Work out the finished part from the listing and answer in its coordinate system (mm). A direction names the side the tool comes from. Coordinates: 2 decimals unless noted, no trailing zeros. Write each loop counter-clockwise with the first axis right and the second up, starting at its lowest first coordinate (ties: lowest second). Pieces come first, ordered by that corner, then holes. Notation, with made-up numbers: (35.5, 13) - (87.5, 13) arc R14 ccw to (87.5, 26) - close; hole circle Ø7 at (42, 88). An arc over 180 degrees is marked (long way). Use one line per item in the form item = value. Start each with the question number.
Item 1: A cutting plane is placed at A-A (x = -11.4). Write down the section's boundary in (y, z) (3 decimals).
Item 2: Given pin 1 (4.5 mm diameter, centred on x = -10.5, z = 5, fed in from +Y); pin 2 (0.9 mm diameter, centred on y = 1, z = 4, fed in from -X); pin 3 (1.5 mm diameter, centred on y = 4, z = -9.5, fed in from +X), each flat-ended and moving along its own axis, determine where each tip first touches the part or whether it passes through.
Item 3: A cutting plane is placed at B-B (z = 9.5). Write down the section's boundary in (x, y).
Item 4: Determine the mould class of faces 3 (the flat face through (-19.6, -2, 0)), 4 (the flat face through (-3.2, -2, 0)), 5 (the flat face through (-9, -3.2, 3)) for opening direction X: released by +X, released by -X, zero draft, split by the parting line, or undercut.
Item 5: Consider probe 1 along X at (y, z) = (-0.85, 0) (3 decimals); probe 2 along Z at (x, y) = (-11.4, -2.6) (3 decimals); probe 3 along X at (y, z) = (-1.3, 0) (3 decimals). Determine where each line is inside the solid, lowest interval first.
Item 6: A cutting plane is placed at C-C (y = 2.75). Write down the section's boundary in (x, z), then the cut area to 3 significant figures.
Item 7: For faces 1 (the flat face through (-7, -0.66, 0)), 2 (the flat face through (-5, 0, 12.7)), determine the directions among +Z, -Z, +X, -X, +Y, -Y from which every point of the face is accessible in a straight line to the end or side of a thin tool.
Item 8: A cutting plane is placed at D-D (z = 1.5). Write down the section's boundary in (x, y), then the cut area to 3 significant figures.
from build123d import *

# Parameters (mm, degrees)
BASE_EXTRUDE_DEPTH = 12.7
SKETCH9_R          = 3.175
CUT_EXTRUDE1_DEPTH = 26.007470884


with BuildPart() as part:
    # Sketch1 → Base-Extrude (new, symmetric)
    with BuildSketch(Plane.XY):
        with BuildLine():
            Line((-14.52, -0.66), (-5.74, -0.66))
            Line((-5.74, -0.66), (-5.74, 0))
            ThreePointArc((-5.74, 0), (0, 5.74), (5.74, 0))
            Line((5.74, 0), (5.74, 1.88))
            ThreePointArc((5.74, 1.88), (7.536051224, -2.456051224), (3.2, -0.66))
            Line((3.2, -0.66), (3.2, 0))
            ThreePointArc((3.2, 0), (0, 3.2), (-3.2, 0))
            Line((-3.2, 0), (-3.2, -3.2))
            Line((-3.2, -3.2), (-19.6, -3.2))
            Line((-19.6, -3.2), (-19.6, -0.66))
            ThreePointArc((-19.6, -0.66), (-17.06, 1.88), (-14.52, -0.66))
        make_face()
    extrude(amount=BASE_EXTRUDE_DEPTH, both=True)

    # Sketch9 → Cut-Extrude1 (cut, through all)
    with BuildSketch(Plane.XZ.offset(3.2)):
        with Locations((-11.4, 0)):
            Circle(SKETCH9_R)
    extrude(amount=-CUT_EXTRUDE1_DEPTH, mode=Mode.SUBTRACT)


solid = part.part
Answer:
q1.outline = (-3.2, -12.7) - (-0.66, -12.7) - (-0.66, -3.175) - (-3.2, -3.175) - close; (-3.2, 3.175) - (-0.66, 3.175) - (-0.66, 12.7) - (-3.2, 12.7) - close
q2.pin_1 = -0.66
q2.pin_2 = -19.29
q2.pin_3 = 4.73
q3.outline = (-19.6, -3.2) - (-3.2, -3.2) - (-3.2, 0) arc R3.2 cw to (3.2, 0) - (3.2, -0.66) arc R2.54 ccw (long way) to (5.74, 1.88) - (5.74, 0) arc R5.74 ccw to (-5.74, 0) - (-5.74, -0.66) - (-14.52, -0.66) arc R2.54 ccw to (-19.6, -0.66) - close
q4.face_3 = released by -X
q4.face_4 = undercut
q4.face_5 = zero draft
q5.probe_1 = -19.6 to -14.575, -8.225 to -3.2, 3.207 to 8.273
q5.probe_2 = -12.7 to -3.175, 3.175 to 12.7
q5.probe_3 = -19.6 to -14.575, -8.225 to -3.2, 3.282 to 8.198
q6.outline = (-5.04, -12.7) - (-1.64, -12.7) - (-1.64, 12.7) - (-5.04, 12.7) - close; (1.64, -12.7) - (5.04, -12.7) - (5.04, 12.7) - (1.64, 12.7) - close
q6.area = 173 mm²
q7.face_1 = +Z, -Z, +Y
q7.face_2 = +Z, +X, -X, +Y, -Y
q8.outline = (-19.6, -3.2) - (-14.2, -3.2) - (-14.2, -0.66) - (-14.52, -0.66) arc R2.54 ccw to (-19.6, -0.66) - close; (-8.6, -3.2) - (-3.2, -3.2) - (-3.2, 0) arc R3.2 cw to (3.2, 0) - (3.2, -0.66) arc R2.54 ccw (long way) to (5.74, 1.88) - (5.74, 0) arc R5.74 ccw to (-5.74, 0) - (-5.74, -0.66) - (-8.6, -0.66) - close
q8.area = 91.8 mm²
